Read the model definition and answer for the solid it produces. Units are mm, in the model's axes. Face numbers are marked on the shaded views. A direction names the side the tool comes from. Coordinates: 2 decimals unless noted, no trailing zeros. Loops run counter-clockwise (first coordinate to the right, second up) from the corner with the lowest first, then second, coordinate; pieces in that order, holes last. Notation, with made-up numbers: M 75,-35.75 L 102,-35.75 A29 cw 102,-12.75 Z; hole C 8,2.25 d7. An arc over 180 degrees is marked long. One line per item, written item: value. Start each with the question number.
1. Flat-ended cylindrical pins translate along their axes: pin 1 (12 mm diameter, centred on x = 4, y = 8, fed in from -Z); pin 2 (1.3 mm diameter, centred on x = 5, z = 14, fed in from +Y); pin 3 (1.3 mm diameter, centred on y = -5, z = 14, fed in from +X). Find the tip coordinate at first contact, or state that the pin passes through.
2. Consider probe 1 along Y at (x, z) = (24, 6); probe 2 along X at (y, z) = (-7, 14.45); probe 3 along X at (y, z) = (-18, 16.5). Determine where each line is inside the solid, lowest interval first.
3. The part is cut by section A-A (z = 14). State how many separate pieces and enclosed holes the cut face has, then the cut area to 3 significant figures.
4. The part is cut by section B-B (z = 8). Write down the section's boundary in (x, y).
5. For the marked faces 1, 2, 3, 4 and 5, determine the directions among +Z, -Z, +X, -X, +Y, -Y from which every point of the face is accessible in a straight line to the end or side of a thin tool.
6. The part is cut by section C-C (y = -17). Write down the section's boundary in (x, z), then the cut area to 3 significant figures.
7. The part is cut by section D-D (x = 7). Write down the section's boundary in (y, z), then the cut area to 3 significant figures.
8. Determine the mould class of the marked faces 6, 7 and 8 for opening direction Y: +Y half, -Y half, draft (parallel to the pull), parting line (faces both ways), or undercut.
```python
from build123d import *

# Parameters (mm, degrees)
STOCK_HORN_ATTACHMENT_START          = 15
STOCK_HORN_ATTACHMENT_PROFILE_R      = 13
STOCK_HORN_ATTACHMENT_DEPTH          = 3
FINGER_ARM_START                     = 15
FINGER_ARM_PROFILE_W                 = 27
FINGER_ARM_PROFILE_H                 = 22
FINGER_ARM_DEPTH                     = 3
DESCENDING_CONTACT_FINGER_PROFILE_W  = 12
DESCENDING_CONTACT_FINGER_PROFILE_H  = 5
DESCENDING_CONTACT_FINGER_DEPTH      = 18
HORN_CENTER_ACCESS_START             = -50
HORN_CENTER_ACCESS_PROFILE_R         = 3
HORN_CENTER_ACCESS_DEPTH             = 89.118237105
CAPTURED_HORN_KEY_BOSS_START         = 13.35
CAPTURED_HORN_KEY_BOSS_PROFILE_R     = 13
CAPTURED_HORN_KEY_BOSS_DEPTH         = 1.65
KEY_POCKET_HUB_START                 = 13.35
STOCK_HORN_POCKET_HUB_R              = 3.55
KEY_POCKET_HUB_DEPTH                 = 1.65
KEY_POCKET_HORIZONTAL_START          = 13.35
STOCK_HORN_POCKET_HORIZONTAL_W       = 16.3
STOCK_HORN_POCKET_HORIZONTAL_H       = 4.2
KEY_POCKET_HORIZONTAL_DEPTH          = 1.65
KEY_POCKET_VERTICAL_START            = 13.35
STOCK_HORN_POCKET_VERTICAL_W         = 4.2
STOCK_HORN_POCKET_VERTICAL_H         = 16.3
KEY_POCKET_VERTICAL_DEPTH            = 1.65
KEY_POCKET_ROUNDED_TIPS_START        = 13.35
STOCK_HORN_POCKET_ROUNDED_TIPS_R     = 2.1
KEY_POCKET_ROUNDED_TIPS_DEPTH        = 1.65
UNMODIFIED_HORN_CAPTURE_M2_START     = -50
UNMODIFIED_HORN_CAPTURE_M2_PROFILE_R = 1.15
UNMODIFIED_HORN_CAPTURE_M2_DEPTH     = 89.118237105
HUB_CLEARANCE_IN_KEY_BOSS_ONLY_START = 13.35
HORN_CENTER_HUB_CLEARANCE_R          = 4
HUB_CLEARANCE_IN_KEY_BOSS_ONLY_DEPTH = 1.65
CONTACT_PAD_KEEPER_START             = -50
CONTACT_PAD_KEEPER_PROFILE_R         = 1.1
CONTACT_PAD_KEEPER_DEPTH             = 89.118237105


with BuildPart() as part:
    # Stock_horn_attachment_profile → Stock_horn_attachment (new body)
    with BuildSketch(Plane.XY.offset(STOCK_HORN_ATTACHMENT_START)):
        Circle(STOCK_HORN_ATTACHMENT_PROFILE_R)
    extrude(amount=STOCK_HORN_ATTACHMENT_DEPTH)

    # Finger_arm_profile → Finger_arm (add)
    with BuildSketch(Plane.XY.offset(FINGER_ARM_START)):
        with Locations((13.5, -8)):
            Rectangle(FINGER_ARM_PROFILE_W, FINGER_ARM_PROFILE_H)
    extrude(amount=FINGER_ARM_DEPTH)

    # Descending_contact_finger_profile → Descending_contact_finger (add)
    with BuildSketch(Plane.XY):
        with Locations((21, -17.5)):
            Rectangle(DESCENDING_CONTACT_FINGER_PROFILE_W, DESCENDING_CONTACT_FINGER_PROFILE_H)
    extrude(amount=DESCENDING_CONTACT_FINGER_DEPTH)

    # Horn_center_access_profile → Horn_center_access (cut, through all)
    with BuildSketch(Plane.XY.offset(HORN_CENTER_ACCESS_START)):
        Circle(HORN_CENTER_ACCESS_PROFILE_R)
    extrude(amount=HORN_CENTER_ACCESS_DEPTH, mode=Mode.SUBTRACT)

    # Captured_horn_key_boss_profile → Captured_horn_key_boss (add)
    with BuildSketch(Plane.XY.offset(CAPTURED_HORN_KEY_BOSS_START)):
        with Locations(Location((0, 0, 0), (0, 0, 270))):
            Circle(CAPTURED_HORN_KEY_BOSS_PROFILE_R)
    extrude(amount=CAPTURED_HORN_KEY_BOSS_DEPTH)

    # Stock_horn_pocket_Hub → Key_pocket_Hub (cut)
    with BuildSketch(Plane.XY.offset(KEY_POCKET_HUB_START)):
        Circle(STOCK_HORN_POCKET_HUB_R)
    extrude(amount=KEY_POCKET_HUB_DEPTH, mode=Mode.SUBTRACT)

    # Stock_horn_pocket_Horizontal → Key_pocket_Horizontal (cut)
    with BuildSketch(Plane.XY.offset(KEY_POCKET_HORIZONTAL_START)):
        Rectangle(STOCK_HORN_POCKET_HORIZONTAL_W, STOCK_HORN_POCKET_HORIZONTAL_H)
    extrude(amount=KEY_POCKET_HORIZONTAL_DEPTH, mode=Mode.SUBTRACT)

    # Stock_horn_pocket_Vertical → Key_pocket_Vertical (cut)
    with BuildSketch(Plane.XY.offset(KEY_POCKET_VERTICAL_START)):
        Rectangle(STOCK_HORN_POCKET_VERTICAL_W, STOCK_HORN_POCKET_VERTICAL_H)
    extrude(amount=KEY_POCKET_VERTICAL_DEPTH, mode=Mode.SUBTRACT)

    # Stock_horn_pocket_Rounded_tips → Key_pocket_Rounded_tips (cut)
    with BuildSketch(Plane.XY.offset(KEY_POCKET_ROUNDED_TIPS_START)):
        with Locations((8.15, 0)):
            Circle(STOCK_HORN_POCKET_ROUNDED_TIPS_R)
        with Locations((-8.15, 0)):
            Circle(STOCK_HORN_POCKET_ROUNDED_TIPS_R)
        with Locations((0, 8.15)):
            Circle(STOCK_HORN_POCKET_ROUNDED_TIPS_R)
        with Locations((0, -8.15)):
            Circle(STOCK_HORN_POCKET_ROUNDED_TIPS_R)
    extrude(amount=KEY_POCKET_ROUNDED_TIPS_DEPTH, mode=Mode.SUBTRACT)

    # Unmodified_horn_capture_M2_profile → Unmodified_horn_capture_M2 (cut, through all)
    with BuildSketch(Plane.XY.offset(UNMODIFIED_HORN_CAPTURE_M2_START)):
        with Locations((7, 7)):
            Circle(UNMODIFIED_HORN_CAPTURE_M2_PROFILE_R)
        with Locations((-7, 7)):
            Circle(UNMODIFIED_HORN_CAPTURE_M2_PROFILE_R)
        with Locations((-7, -7)):
            Circle(UNMODIFIED_HORN_CAPTURE_M2_PROFILE_R)
        with Locations((7, -7)):
            Circle(UNMODIFIED_HORN_CAPTURE_M2_PROFILE_R)
    extrude(amount=UNMODIFIED_HORN_CAPTURE_M2_DEPTH, mode=Mode.SUBTRACT)

    # Horn_center_hub_clearance → Hub_clearance_in_key_boss_only (cut)
    with BuildSketch(Plane.XY.offset(HUB_CLEARANCE_IN_KEY_BOSS_ONLY_START)):
        Circle(HORN_CENTER_HUB_CLEARANCE_R)
    extrude(amount=HUB_CLEARANCE_IN_KEY_BOSS_ONLY_DEPTH, mode=Mode.SUBTRACT)

    # Contact_pad_keeper_profile → Contact_pad_keeper (cut, through all)
    with BuildSketch(Plane.XY.offset(CONTACT_PAD_KEEPER_START)):
        with Locations(Location((18, -17.5, 0), (0, 0, 180))):
            Circle(CONTACT_PAD_KEEPER_PROFILE_R)
        with Locations(Location((24, -17.5, 0), (0, 0, 180))):
            Circle(CONTACT_PAD_KEEPER_PROFILE_R)
    extrude(amount=CONTACT_PAD_KEEPER_DEPTH, mode=Mode.SUBTRACT)


solid = part.part
```
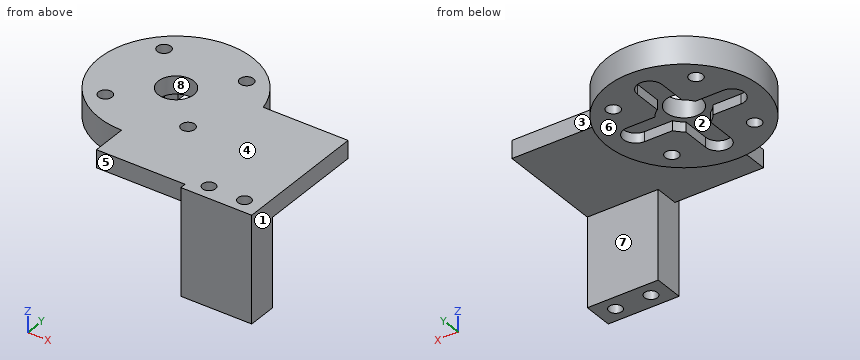
Answer block:
1. pin 1: stops at z = 13.35
1. pin 2: stops at y = 12.25
1. pin 3: stops at x = 12.25
2. probe 1: y = -20 to -18.6, -16.4 to -15
2. probe 2: x = -10.95 to -8.15, -5.85 to -2.1, 2.1 to 5.85, 8.15 to 10.95
2. probe 3: x = 0 to 17.02, 18.98 to 23.02, 24.98 to 27
3. separate pieces: 2
3. enclosed holes: 7
3. area: 416 mm2
4. outline: M 15,-20 L 27,-20 L 27,-15 L 15,-15 Z; hole C 18,-17.5 d2.2; hole C 24,-17.5 d2.2
5. face 1: +Z, -Z, +X, +Y, -Y
5. face 2: -Z
5. face 3: +Z, -Z, +X, +Y
5. face 4: +Z, +X, -X, +Y, -Y
5. face 5: +Z, -Z, -X, -Y
6. outline: M 0,15 L 15,15 L 15,0 L 17.02,0 L 17.02,18 L 0,18 Z; M 18.98,0 L 23.02,0 L 23.02,18 L 18.98,18 Z; M 24.98,0 L 27,0 L 27,18 L 24.98,18 Z
6. area: 190 mm2
7. outline: M -19,15 L -10.95,15 L -10.95,13.35 L -8.15,13.35 L -8.15,18 L -19,18 Z; M -5.85,13.35 L -2.1,13.35 L -2.1,15 L 2.1,15 L 2.1,13.35 L 5.85,13.35 L 5.85,18 L -5.85,18 Z; M 8.15,13.35 L 10.95,13.35 L 10.95,18 L 8.15,18 Z
7. area: 97.7 mm2
8. face 6: draft
8. face 7: +Y half
8. face 8: undercut
